```python
from build123d import *

# Parameters (mm, degrees)
F0_W     = 48.771314
F0_H     = 45.987077
F1_DEPTH = 50
F2_SIZE  = 5
F3_R     = 4.711226
F4_DEPTH = 50.001


with BuildPart() as f1:
    # F0 (on Front) → F1 (new body)
    with BuildSketch(Plane.XZ):
        with Locations((24.385657, 22.993538)):
            Rectangle(F0_W, F0_H)
    extrude(amount=F1_DEPTH)

    # F2
    f2_edges = [f1.edges().sort_by_distance(p)[0] for p in [
        (0, -50, 22.993539),
        (24.385657, -50, 0),
        (48.771314, -50, 22.993539),
        (24.385657, -50, 45.987077),
        (48.771314, -25, 0),
        (48.771314, -25, 45.987077),
        (48.771314, 0, 22.993539),
        (0, -25, 45.987077),
        (24.385657, 0, 45.987077),
        (0, -25, 0),
        (24.385657, 0, 0),
        (0, 0, 22.993539),
    ]]
    chamfer(f2_edges, length=F2_SIZE)

    # F3 (on face) → F4 (cut, through all)
    with BuildSketch(Plane(origin=(0, 0, 0), x_dir=(-1, 0, 0), z_dir=(0, 1, 0))):
        with Locations((-26.383946, 24.235671)):
            Circle(F3_R)
    extrude(amount=-F4_DEPTH, mode=Mode.SUBTRACT)


solid = f1.part
```
Input: part model. Units: mm. Frame: model coordinates. Give positions to 0.01 mm unless a question says otherwise; leave off trailing zeros. Order: outer loops, then holes, each group sorted by start corner. A loop starts at its lowest first (then second) coordinate and runs counter-clockwise, first axis right, second up. Notation, with made-up numbers: M 81.5,8.5 L 96.5,8.5 A8 ccw 96.5,12.5 Z; hole C 38,35 d6. An arc over 180 degrees is marked long. Return JSON: item names as keys, results as strings.
1) Mould query, pull axis X, two halves, no side actions, for faces 1 (the face through (24, -25, 45.987)), 2 (the face through (29.856, -24.65, 27.42)), 3 (the face through (2.535, -24.72, 43.522)). Classes: released by +X, released by -X, zero draft, split by the parting line, or undercut.
Taken from the geometry:
{"face 1": "zero draft", "face 2": "undercut", "face 3": "released by -X"}
2) Line query: L1, parallel to X at y = -34.5, z = 23.5; L2, parallel to X at y = -13, z = 21.5; L3, parallel to Y at x = 27, z = 2. Output: solid intervals per line, ascending. Write a range as [from, to].
Taken from the geometry:
{"L1": "x = [0, 21.73], [31.04, 48.77]", "L2": "x = [0, 22.55], [30.22, 48.77]", "L3": "y = [-47, -3]"}
3) Section query A-A on z = 10. Output: boundary loops of the cut face in (x, y).
Taken from the geometry:
{"outline": "M 0,-45 L 5,-50 L 43.77,-50 L 48.77,-45 L 48.77,-5 L 43.77,0 L 5,0 L 0,-5 Z"}
4) Section query D-D on z = 25. Output: boundary loops of the cut face in (x, y).
Taken from the geometry:
{"outline": "M 0,-45 L 5,-50 L 21.74,-50 L 21.74,0 L 5,0 L 0,-5 Z; M 31.03,-50 L 43.77,-50 L 48.77,-45 L 48.77,-5 L 43.77,0 L 31.03,0 Z"}
5) Section query C-C on y = -30. Output: boundary loops of the cut face in (x, z).
Taken from the geometry:
{"outline": "M 0,5 L 5,0 L 43.77,0 L 48.77,5 L 48.77,40.99 L 43.77,45.99 L 5,45.99 L 0,40.99 Z; hole C 26.38,24.24 d9.42"}
6) Section query B-B on x = 29.5. Output: boundary loops of the cut face in (y, z), and give its area (3 significant figures).
Taken from the geometry:
{"outline": "M -50,5 L -45,0 L -5,0 L 0,5 L 0,20.7 L -50,20.7 Z; M -50,27.77 L 0,27.77 L 0,40.99 L -5,45.99 L -45,45.99 L -50,40.99 Z", "area": "1,900 mm2"}
